```python
from build123d import *

# Parameters (mm, degrees)
F3_R     = 3.2
F4_DEPTH = 18
F5_COUNT = 8


with BuildPart() as f2:
    # F1 (on Front) → F2 (revolve)
    with BuildSketch(Plane.XZ):
        Polygon((0, 75), (0, 47), (18, 47), (18, 48.5), (8, 48.5), (8, 57.5), (18, 57.5), (18, 75), align=None)
    revolve(axis=Axis((9, 0, 0), (1, 0, 0)))


with BuildPart() as f4:
    # F3 (on face) → F4 (new body, through all)
    with BuildSketch(Plane.YZ.offset(18)):
        with Locations((0, 65)):
            Circle(F3_R)
    extrude(amount=-F4_DEPTH)


with BuildPart() as f5_1:
    # F5: instance of F4
    add(f4.part.rotate(Axis((18, 0, 0), (1, 0, 0)), 1 * 360 / F5_COUNT))


with BuildPart() as f5_2:
    # F5: instance of F4
    add(f4.part.rotate(Axis((18, 0, 0), (1, 0, 0)), 2 * 360 / F5_COUNT))


with BuildPart() as f5_3:
    # F5: instance of F4
    add(f4.part.rotate(Axis((18, 0, 0), (1, 0, 0)), 3 * 360 / F5_COUNT))


with BuildPart() as f5_4:
    # F5: instance of F4
    add(f4.part.rotate(Axis((18, 0, 0), (1, 0, 0)), 4 * 360 / F5_COUNT))


with BuildPart() as f5_5:
    # F5: instance of F4
    add(f4.part.rotate(Axis((18, 0, 0), (1, 0, 0)), 5 * 360 / F5_COUNT))


with BuildPart() as f5_6:
    # F5: instance of F4
    add(f4.part.rotate(Axis((18, 0, 0), (1, 0, 0)), 6 * 360 / F5_COUNT))


with BuildPart() as f5_7:
    # F5: instance of F4
    add(f4.part.rotate(Axis((18, 0, 0), (1, 0, 0)), 7 * 360 / F5_COUNT))


with BuildPart() as f2_1:
    add(f2.part)

    # F6: cut F4, F5_1, F5_2, F5_3, F5_4, F5_5, F5_6, F5_7
    add(f4.part, mode=Mode.SUBTRACT)
    add(f5_1.part, mode=Mode.SUBTRACT)
    add(f5_2.part, mode=Mode.SUBTRACT)
    add(f5_3.part, mode=Mode.SUBTRACT)
    add(f5_4.part, mode=Mode.SUBTRACT)
    add(f5_5.part, mode=Mode.SUBTRACT)
    add(f5_6.part, mode=Mode.SUBTRACT)
    add(f5_7.part, mode=Mode.SUBTRACT)


solid = f2_1.part
```
Can you work these out from the model? Positions are in its coordinate system, mm. A direction names the side the tool comes from. Give positions to 0.01 mm unless a question says otherwise; leave off trailing zeros. Order: outer loops, then holes, each group sorted by start corner. A loop starts at its lowest first (then second) coordinate and runs counter-clockwise, first axis right, second up. Notation, with made-up numbers: (11, 82) - (69, 82) arc R24 ccw to (69, 114) - close; hole circle Ø2 at (9.25, 70). An arc over 180 degrees is marked (long way). Use a Markdown table: item, result. Add a question column.
Q1. I'm going to push flat-ended pins straight in: pin 1 (5 mm diameter, centred on x = 8.5, z = -46, fed in from -Y); pin 2 (8.5 mm diameter, centred on y = -45.96, z = -45.96, fed in from +X); pin 3 (4 mm diameter, centred on x = 5.5, z = -17.5, fed in from +Y); pin 4 (1.5 mm diameter, centred on x = 12.5, z = 31, fed in from +Y). Where does each tip first touch, or does it pass through?
Q2. Please list where these lines run through material, in increasing order: line 1 along Z through (x, y) = (13.5, 0.5); line 2 along Z through (x, y) = (13, -24); line 3 along Z through (x, y) = (16.25, 33).
Q3. If we section it at A-A on x = 11: Count the separate pieces of the cut face and the enclosed holes in it, plus the area to 3 significant figures.
Q4. If we mould it in two halves opening along Y, with no side actions, what happens to faces 1 (the cylindrical face through (9.126, 61.876, 0.694)), 2 (the cylindrical face through (8.874, -74.362, -9.764)), 3 (the flat face through (18, -40, 25))? For each: released by +Y, released by -Y, zero draft, split by the parting line, or undercut.
Q5. If we section it at D-D on z = 65: Write out the boundary of the cut face in (x, y).
Q6. On a 3-axis mill with a long thin cutter (end or side, diameter ignored), from which of +Z, -Z, +X, -X, +Y, -Y can I reach the whole of each face in a straight line? I mean faces 4 (the cylindrical face through (9.126, 0.694, -61.876)), 5 (the cylindrical face through (13.07, 56.133, -12.465)). Say none if no direction works.
Q7. If we section it at B-B on y = 0: Write out the boundary of the cut face in (x, z), plus the area to 3 significant figures.
Answers follow:
| question | item | result |
|---|---|---|
| 1 | pin 1 | stops at y = -61.1 |
| 1 | pin 2 | stops at x = 18 |
| 1 | pin 3 | stops at y = 73.38 |
| 1 | pin 4 | stops at y = 68.63 |
| 2 | line 1 | z = -75 to -68.16, -61.84 to -57.5, -48.5 to -47, 47 to 48.5, 57.5 to 61.84, 68.16 to 75 |
| 2 | line 2 | z = -71.06 to -52.25, -42.15 to -40.41, 40.41 to 42.15, 52.25 to 71.06 |
| 2 | line 3 | z = -67.35 to -47.09, -35.54 to -33.47, 33.47 to 35.54, 47.09 to 67.35 |
| 3 | separate pieces | 2 |
| 3 | enclosed holes | 10 |
| 3 | area | 7,480 mm^2 |
| 4 | face 1 | undercut |
| 4 | face 2 | split by the parting line |
| 4 | face 3 | zero draft |
| 5 | outline | (0, -37.42) - (18, -37.42) - (18, -3.2) - (0, -3.2) - close; (0, 3.2) - (18, 3.2) - (18, 37.42) - (0, 37.42) - close |
| 6 | face 4 | +X, -X |
| 6 | face 5 | +X |
| 7 | outline | (0, -75) - (18, -75) - (18, -68.2) - (0, -68.2) - close; (0, -61.8) - (18, -61.8) - (18, -57.5) - (8, -57.5) - (8, -48.5) - (18, -48.5) - (18, -47) - (0, -47) - close; (0, 47) - (18, 47) - (18, 48.5) - (8, 48.5) - (8, 57.5) - (18, 57.5) - (18, 61.8) - (0, 61.8) - close; (0, 68.2) - (18, 68.2) - (18, 75) - (0, 75) - close |
| 7 | area | 598 mm^2 |
